Check sheet for the drawn part. Datum: minimum x, y, z corner. Units: mm. Give positions to 0.01 mm unless a question says otherwise; leave off trailing zeros. Order: outer loops, then holes, each group sorted by start corner. A loop starts at its lowest first (then second) coordinate and runs counter-clockwise, first axis right, second up.
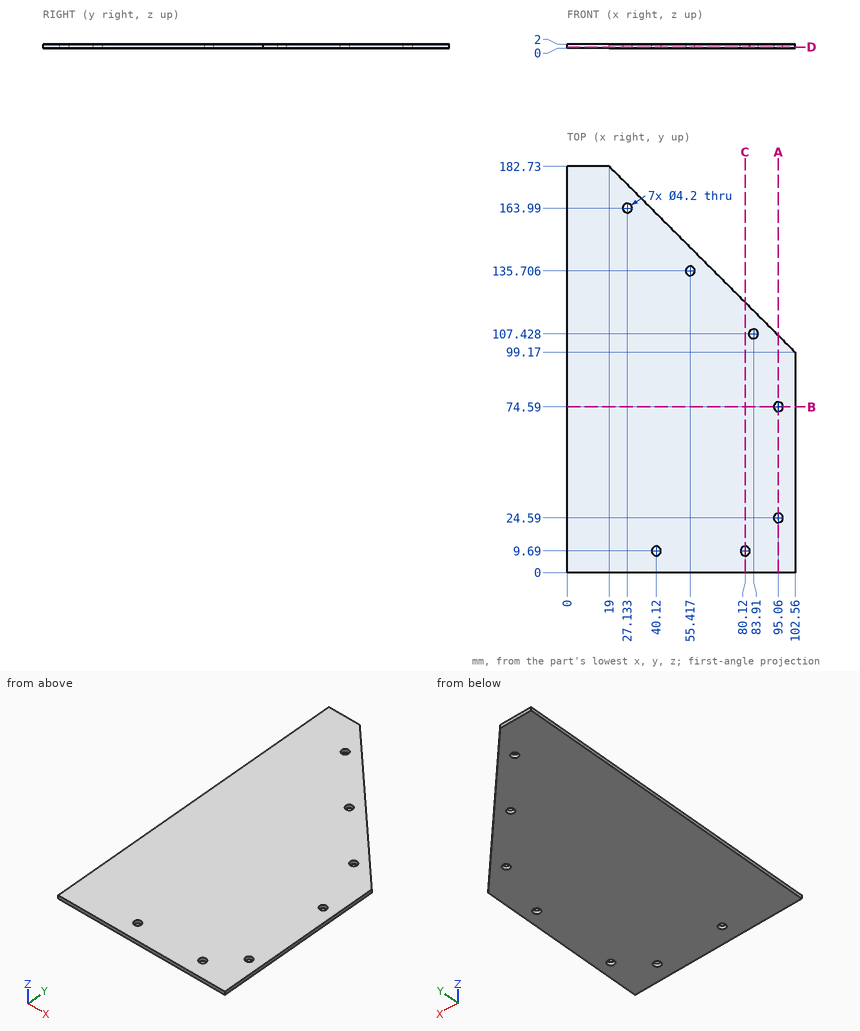
Q1. Sectioned sample at D-D, the plane z = 0.6. Record the cut outline in (x, y), plus the area to 3 significant figures.
Q2. Material ranges on line 1 (Y direction, x = 95.06, z = 0.95); line 2 (X direction, y = 106, z = 1.05); line 3 (X direction, y = 8, z = 1.55) (1 decimal), recorded low to high.
Q3. Sectioned sample at C-C, the plane x = 80.12. Record the cut outline in (y, z).
Q4. Sectioned sample at A-A, the plane x = 95.06. Record the cut outline in (y, z).
Q5. Sectioned sample at B-B, the plane y = 74.59. Record the cut outline in (x, z), plus the area to 3 significant figures.
Filled in:
1. outline: (0, 0) - (102.56, 0) - (102.56, 99.17) - (19, 182.73) - (0, 182.73) - close; hole circle Ø4.2 at (27.13, 163.99); hole circle Ø4.2 at (40.12, 9.69); hole circle Ø4.2 at (55.42, 135.71); hole circle Ø4.2 at (80.12, 9.69); hole circle Ø4.2 at (83.91, 107.43); hole circle Ø4.2 at (95.06, 24.59); hole circle Ø4.2 at (95.06, 74.59)
1. area: 15,200 mm2
2. line 1: y = 0 to 22.49, 26.69 to 72.49, 76.69 to 106.67
2. line 2: x = 0 to 82.37, 85.45 to 95.73
2. line 3: x = 0 to 38.9, 41.4 to 78.9, 81.4 to 102.6
3. outline: (0, 0) - (7.59, 0) - (7.59, 2) - (0, 2) - close; (11.79, 0) - (121.61, 0) - (121.61, 2) - (11.79, 2) - close
4. outline: (0, 0) - (22.49, 0) - (22.49, 2) - (0, 2) - close; (26.69, 0) - (72.49, 0) - (72.49, 2) - (26.69, 2) - close; (76.69, 0) - (106.67, 0) - (106.67, 2) - (76.69, 2) - close
5. outline: (0, 0) - (92.96, 0) - (92.96, 2) - (0, 2) - close; (97.16, 0) - (102.56, 0) - (102.56, 2) - (97.16, 2) - close
5. area: 197 mm2
